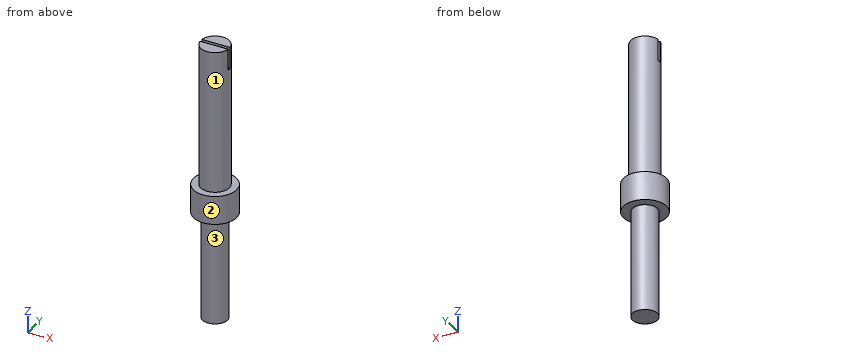
from build123d import *

# Parameters (mm, degrees)
SKETCH_1_R          = 3
EXTRUDE_1_DEPTH     = 4
SKETCH_2_R          = 2
EXTRUDE_2_DEPTH     = 20
SKETCH_3_R          = 1.75
EXTRUDE_3_DEPTH     = 15
SKETCH_4_W          = 4.461198183
SKETCH_4_H          = 0.5
CUT_EXTRUDE_1_DEPTH = 3


with BuildPart() as part:
    # 스케치1 → 보스-돌출1 (new body)
    with BuildSketch(Plane.XY):
        Circle(SKETCH_1_R)
    extrude(amount=EXTRUDE_1_DEPTH)

    # 스케치2 → 보스-돌출2 (add)
    with BuildSketch(Plane.XY.offset(4)):
        Circle(SKETCH_2_R)
    extrude(amount=EXTRUDE_2_DEPTH)

    # 스케치3 → 보스-돌출3 (add)
    with BuildSketch(Plane(origin=(0, 0, 0), x_dir=(-1, 0, 0), z_dir=(0, 0, -1))):
        Circle(SKETCH_3_R)
    extrude(amount=EXTRUDE_3_DEPTH)

    # 스케치4 → 컷-돌출1 (cut)
    with BuildSketch(Plane.XY.offset(24)):
        with Locations((-0.011637909, 0)):
            Rectangle(SKETCH_4_W, SKETCH_4_H)
    extrude(amount=-CUT_EXTRUDE_1_DEPTH, mode=Mode.SUBTRACT)


solid = part.part
The listing builds one solid part. Answer for the finished solid, in the listing's coordinates (mm). Face numbers are marked on the shaded views. A direction names the side the tool comes from. Coordinates: 2 decimals unless noted, no trailing zeros. Order: outer loops, then holes, each group sorted by start corner. A loop starts at its lowest first (then second) coordinate and runs counter-clockwise, first axis right, second up. Notation, with made-up numbers: (-12, 82.5) -> (46, 82.5) arc R17 cw to (46, 96.5) -> close; hole circle Ø10 at (84, -40). An arc over 180 degrees is marked (long way). Answer in a Markdown table with one row per item. Add a question column.
Item 1: Which of the six approach directions +Z, -Z, +X, -X, +Y, -Y give full straight-line access (tool end or side, diameter ignored) to the marked faces 1, 2 and 3?
Item 2: Each of these flat-tipped pins is pushed along its axis until it touches: P1, Ø2, axis at x = -2.5, z = 0, coming from the -Y side; P2, Ø3, axis at x = 1, z = -2, coming from the -Y side; P3, Ø3.5, axis at x = -1, z = 22, coming from the -Y side. Where does it stop, or does it pass through?
Item 3: Find section A-A (x = 0). Write down the section's boundary in (y, z), then the cut area to 3 significant figures.
Item 4: Find section B-B (y = -0.6). Write down the section's boundary in (x, z).
Item 5: Find section D-D (z = -10.5). Write down the section's boundary in (x, y), then the cut area to 3 significant figures.
Item 6: Find the intervals of material crossed by L1, parallel to Z at x = 1.9, y = -0.9; L2, parallel to X at y = 0.05, z = 14; L3, parallel to Z at x = -1.5, y = 1.2, in increasing order. Write a range as from..to.
Item 7: Find section C-C (z = 16.5). Write down the section's boundary in (x, y), then the cut area to 3 significant figures.
Result set:
| question | item | result |
|---|---|---|
| 1 | face 1 | +Z |
| 1 | face 2 | +Z, -Z |
| 1 | face 3 | -Z |
| 2 | P1 | stops at y = -2.6 |
| 2 | P2 | stops at y = -1.75 |
| 2 | P3 | stops at y = -2 |
| 3 | outline | (-3, 0) -> (-1.75, 0) -> (-1.75, -15) -> (1.75, -15) -> (1.75, 0) -> (3, 0) -> (3, 4) -> (2, 4) -> (2, 24) -> (0.25, 24) -> (0.25, 21) -> (-0.25, 21) -> (-0.25, 24) -> (-2, 24) -> (-2, 4) -> (-3, 4) -> close |
| 3 | area | 155 mm² |
| 4 | outline | (-2.94, 0) -> (-1.64, 0) -> (-1.64, -15) -> (1.64, -15) -> (1.64, 0) -> (2.94, 0) -> (2.94, 4) -> (1.91, 4) -> (1.91, 24) -> (-1.91, 24) -> (-1.91, 4) -> (-2.94, 4) -> close |
| 5 | outline | circle Ø3.5 at (0, 0) |
| 5 | area | 9.62 mm² |
| 6 | L1 | z = 0..4 |
| 6 | L2 | x = -2..2 |
| 6 | L3 | z = 0..24 |
| 7 | outline | circle Ø4 at (0, 0) |
| 7 | area | 12.6 mm² |
